The drawing under review shows one solid part. Ordinate dimensions are in mm from its lowest x, y, z. Give positions to 0.01 mm unless a question says otherwise; leave off trailing zeros. Order: outer loops, then holes, each group sorted by start corner. A loop starts at its lowest first (then second) coordinate and runs counter-clockwise, first axis right, second up. Notation, with made-up numbers: (11.25, 27) - (68.25, 27) arc R30 ccw to (68.25, 55) - close; hole circle Ø2 at (-33, 39). An arc over 180 degrees is marked (long way). Write item = value, one per line. Start each with the question number.
1. We need section B-B, the plane y = 4. Give the boundary of the cut face in (x, z), and give its area (3 significant figures).
2. Wall thickness on probe 1 along X at (y, z) = (4.5, 130) (1 decimal); probe 2 along Z at (x, y) = (174, 6.25) (1 decimal); probe 3 along X at (y, z) = (2, 128): over which ranges is each line inside the solid? List them lowest first.
3. We need section A-A, the plane x = 125. Give the boundary of the cut face in (y, z).
4. We need section C-C, the plane z = 150. Give the boundary of the cut face in (x, y).
5. For P1, Ø4, axis at x = 168.5, y = 6, coming from the +Z side (1 decimal); P2, Ø2, axis at y = 7, z = 153.5, coming from the -X side (1 decimal); P3, Ø4, axis at x = 194.5, y = 8.5, coming from the +Z side, all flat-tipped, find the tip position at first contact; note any pin that passes through.
6. We need section D-D, the plane x = 232. Give the boundary of the cut face in (y, z), and give its area (3 significant figures).
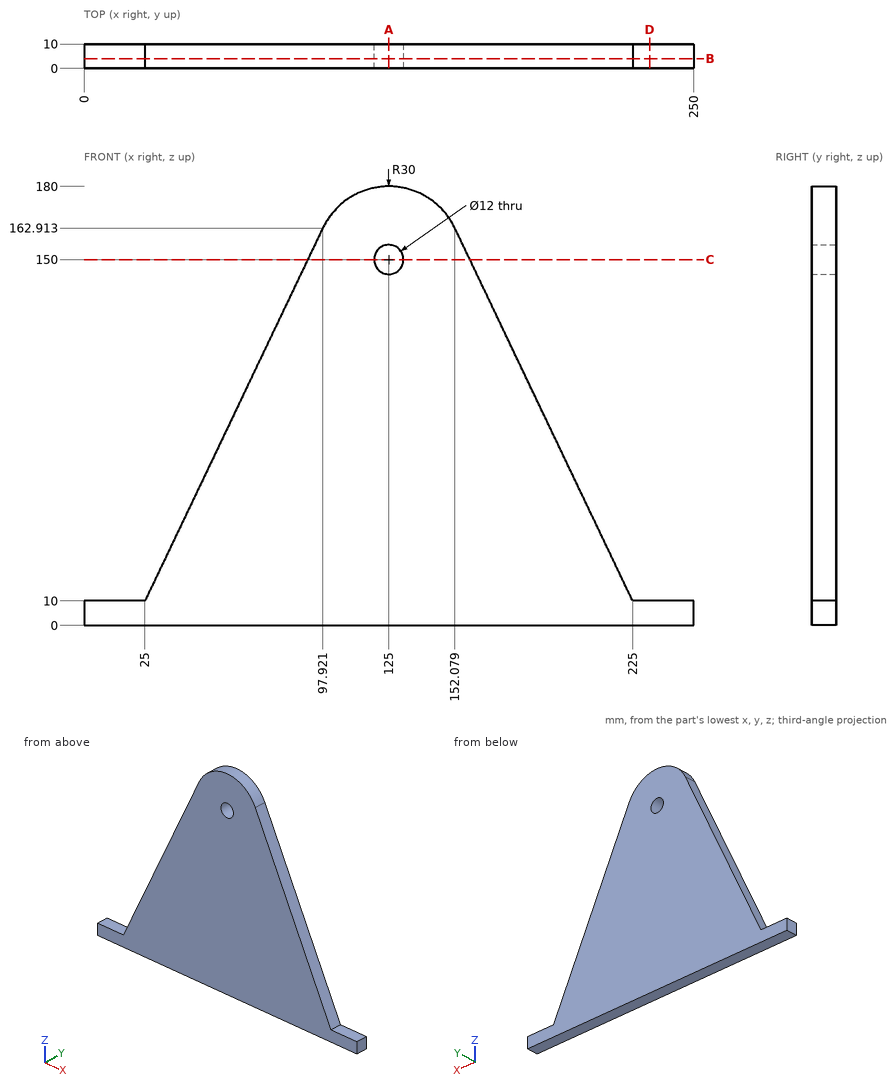
Model answer:
q1.outline = (0, 0) - (250, 0) - (250, 10) - (225, 10) - (152.08, 162.91) arc R30 ccw to (97.92, 162.91) - (25, 10) - (0, 10) - close; hole circle Ø12 at (125, 150)
q1.area = 22,500 mm2
q2.probe_1 = 82.2 to 167.8
q2.probe_2 = 0 to 116.9
q2.probe_3 = 81.27 to 168.73
q3.outline = (0, 0) - (10, 0) - (10, 144) - (0, 144) - close; (0, 156) - (10, 156) - (10, 180) - (0, 180) - close
q4.outline = (91.76, 0) - (119, 0) - (119, 10) - (91.76, 10) - close; (131, 0) - (158.24, 0) - (158.24, 10) - (131, 10) - close
q5.P1 = 132.7
q5.P2 = 93
q5.P3 = 78.15
q6.outline = (0, 0) - (10, 0) - (10, 10) - (0, 10) - close
q6.area = 100 mm2
